Could you check a few things on this model? Use its own coordinates, in mm. A direction names the side the tool comes from. Give positions to 0.01 mm unless a question says otherwise; leave off trailing zeros. Loops run counter-clockwise (first coordinate to the right, second up) from the corner with the lowest first, then second, coordinate; pieces in that order, holes last.
1. I need wall thicknesses on line 1 along X through (y, z) = (21.75, 21). Which ranges of the line are inside material? Lowest first, please.
2. For P1, Ø2, axis at y = 4.5, z = -14.5, coming from the +X side; P2, Ø7.5, axis at x = -57.5, z = 8.5, coming from the +Y side; P3, Ø2, axis at y = 18.5, z = -5.5, coming from the -X side, each with a flat end and sliding along its axis, tell me the tip position at first contact or that it passes through.
3. Imagine slicing it at B-B (y = 12.5). List the corners of the cut face in (x, z) for me, plus the area to 4 significant figures.
4. Thinking about a two-plate mould opening in Z: for faces 5 (the flat face through (-56, 3, 9)), 6 (the flat face through (-1, 15, 32.5)), 7 (the flat face through (56.738, 1.479, -6.014)), which applies, +Z half, -Z half, draft (parallel to the pull), parting line (faces both ways), or undercut?
5. Imagine slicing it at A-A (z = -15). List the corners of the cut face in (x, y) for me, plus the area to 3 significant figures.
6. For faces 1 (the flat face through (-56.738, 1.479, 6.014)), 2 (the flat face through (56, 3, -9)), 3 (the flat face through (-56, 3, -9)), 4 (the flat face through (-56.621, 1.479, 11.014)), which set-ups out of +Z, -Z, +X, -X, +Y, -Y let a thin tool reach every point of the face, with its end or its side?
```python
from build123d import *

# Parameters (mm, degrees)
SKETCH1_W            = 105
SKETCH1_H            = 65
BOSS_EXTRUDE1_DEPTH  = 30
BOSS_EXTRUDE2_DEPTH  = 3
MIRROR2_COPY_1_DEPTH = 3


with BuildPart() as part:
    # Sketch1 → Boss-Extrude1 (new body)
    with BuildSketch(Plane(origin=(0, 0, 0), x_dir=(1, 0, 0), z_dir=(0, 1, 0))):
        Rectangle(SKETCH1_W, SKETCH1_H)
    extrude(amount=BOSS_EXTRUDE1_DEPTH)

    # Sketch3 → Boss-Extrude2 (add)
    with BuildSketch(Plane.XZ):
        with BuildLine():
            Line((52.5, 12), (60.858898944, 10))
            ThreePointArc((60.858898944, 10), (62.042338631, 8.5), (60.858898944, 7))
            Line((60.858898944, 7), (52.5, 5))
            Line((52.5, 5), (52.5, 12))
        make_face()
    boss_extrude2 = extrude(amount=-BOSS_EXTRUDE2_DEPTH)

    # Mirror1: Boss-Extrude2 across plane
    add(boss_extrude2.mirror(Plane.XY))

    # Mirror2: Boss-Extrude2 across plane
    add(boss_extrude2.mirror(Plane(origin=(0, 0, 0), x_dir=(0, 0, 1), z_dir=(1, 0, 0))))

    # Mirror2 copy 1 sketch → Mirror2 copy 1 (add)
    with BuildSketch(Plane(origin=(0, 0, 0), x_dir=(-1, 0, 0), z_dir=(0, -1, 0))):
        with BuildLine():
            Line((52.5, 12), (60.858898944, 10))
            ThreePointArc((60.858898944, 10), (62.042338631, 8.5), (60.858898944, 7))
            Line((60.858898944, 7), (52.5, 5))
            Line((52.5, 5), (52.5, 12))
        make_face()
    extrude(amount=-MIRROR2_COPY_1_DEPTH)


solid = part.part
```
Derived:
1. line 1: x = -52.5 to 52.5
2. P1: stops at x = 52.5
2. P2: stops at y = 3
2. P3: stops at x = -52.5
3. outline: (-52.5, -32.5) - (52.5, -32.5) - (52.5, 32.5) - (-52.5, 32.5) - close
3. area: 6,825 mm2
4. face 5: draft
4. face 6: +Z half
4. face 7: undercut
5. outline: (-52.5, 0) - (52.5, 0) - (52.5, 30) - (-52.5, 30) - close
5. area: 3,150 mm2
6. face 1: -X, +Y, -Y
6. face 2: +Z, -Z, +X, +Y
6. face 3: +Z, -Z, -X, +Y
6. face 4: +Z, -X, +Y, -Y
